```python
from build123d import *

# Parameters (mm, degrees)
F0_W     = 93.4585928917
F0_H     = 52.6832342148
F1_DEPTH = 5
F3_DEPTH = 52.6832342148


# Not quite as in the source:
# - a feature names something its author has since deleted; it is built from what else it names


with BuildPart() as f1:
    # F0 (on Top) → F1 (new body)
    with BuildSketch(Plane.XY):
        Rectangle(F0_W, F0_H)
    extrude(amount=F1_DEPTH)

    # F2 (on face) → F3 (join, through all)
    with BuildSketch(Plane.XZ.offset(26.3416171074)):
        with BuildLine():
            ThreePointArc((-46.7292964458, -8.8555142283), (-44.1355763793, -2.5937200666), (-37.8737822175, 0))
            Line((-37.8737822175, 0), (-46.7292964458, 0))
            Line((-46.7292964458, 0), (-46.7292964458, -8.8555142283))
        make_face()
        with BuildLine():
            ThreePointArc((46.7292964458, -8.8555142283), (44.1355763793, -2.5937200666), (37.8737822175, 0))
            ThreePointArc((37.8737822175, 0), (31.6119880557, -15.1173083901), (46.7292964458, -8.8555142283))
        make_face()
        with BuildLine():
            ThreePointArc((-46.7292964458, -8.8555142283), (-37.8737822175, -17.7110284567), (-29.0182679892, -8.8555142283))
            ThreePointArc((-29.0182679892, -8.8555142283), (-31.6119880557, -2.5937200666), (-37.8737822175, 0))
            ThreePointArc((-37.8737822175, 0), (-44.1355763793, -2.5937200666), (-46.7292964458, -8.8555142283))
        make_face()
        with BuildLine():
            Line((46.7292964458, 0), (37.8737822175, 0))
            ThreePointArc((37.8737822175, 0), (44.1355763793, -2.5937200666), (46.7292964458, -8.8555142283))
            Line((46.7292964458, -8.8555142283), (46.7292964458, 0))
        make_face()
    extrude(amount=-F3_DEPTH)


solid = f1.part
```
Read the model definition and answer for the solid it produces. Units are mm, in the model's axes. Give positions to 0.01 mm unless a question says otherwise; leave off trailing zeros. Write each loop counter-clockwise with the first axis right and the second up, starting at its lowest first coordinate (ties: lowest second). Pieces come first, ordered by that corner, then holes. Notation, with made-up numbers: M -38.5,-8 L 17.5,-8 A15 cw 17.5,21 Z; hole C -9,60 d7. An arc over 180 degrees is marked long. Put each result on its own line as item: value. Start each with the question number.
1. The part is cut by section D-D, the plane x = 11. Give the vertices of the cut face in (y, z).
2. For a pull along Z with two mould halves and no side action, classify faces 1 (the flat face through (46.729, 0, -2)), 2 (the flat face through (-1, 0, 0)), 3 (the flat face through (-1, 0, 5)) as released by +Z, released by -Z, zero draft, split by the parting line, or undercut.
3. The part is cut by section C-C, the plane y = 17.5. Give the vertices of the cut face in (x, z), and give its area (3 significant figures).
4. Consider line 1 along X through (y, z) = (20, -8.5); line 2 along Z through (x, y) = (13, 8); line 3 along X through (y, z) = (-10.5, -15.75). Determine where each line is inside the solid, lowest interval first.
5. The part is cut by section B-B, the plane x = -33. Give the vertices of the cut face in (y, z).
6. Each of these flat-tipped pins is pushed along its axis until it touches: pin 1 Ø4 at (x, y) = (-33, 3) entering from -Z; pin 2 Ø8 at (x, y) = (-14, -4.5) entering from -Z. Where does it stop, or does it pass through?
7. The part is cut by section A-A, the plane z = -3.75. Give the vertices of the cut face in (x, y).
Final values:
1. outline: M -26.34,0 L 26.34,0 L 26.34,5 L -26.34,5 Z
2. face 1: zero draft
2. face 2: undercut
2. face 3: released by +Z
3. outline: M -46.73,-8.86 A8.86 ccw long -37.87,0 L 37.87,0 A8.86 ccw long 46.73,-8.86 L 46.73,5 L -46.73,5 Z
3. area: 994 mm²
4. line 1: x = -46.73 to -29.03, 29.03 to 46.73
4. line 2: z = 0 to 5
4. line 3: x = -43.43 to -32.32, 32.32 to 43.43
5. outline: M -26.34,-16.25 L 26.34,-16.25 L 26.34,-1.46 L -26.34,-1.46 Z; M -26.34,0 L 26.34,0 L 26.34,5 L -26.34,5 Z
6. pin 1: stops at z = -17.23
6. pin 2: stops at z = 0
7. outline: M -46.73,-26.34 L -30.64,-26.34 L -30.64,26.34 L -46.73,26.34 Z; M 30.64,-26.34 L 46.73,-26.34 L 46.73,26.34 L 30.64,26.34 Z
